from build123d import *

# Parameters (mm, degrees)
SKETCH_1_R          = 5
EXTRUDE_1_DEPTH     = 10
SKETCH_2_R          = 5
EXTRUDE_2_DEPTH     = 20
SKETCH_3_R          = 2.5
CUT_EXTRUDE_1_DEPTH = 15
SKETCH_4_R          = 2.5
CUT_EXTRUDE_2_DEPTH = 29.722813233


with BuildPart() as part:
    # 草圖1 → 填料-伸長1 (new, symmetric)
    with BuildSketch(Plane(origin=(0, 0, 0), x_dir=(1, 0, 0), z_dir=(0, 1, 0))):
        with Locations(Location((0, 0, 0), (0, 0, 270))):
            Circle(SKETCH_1_R)
    extrude(amount=EXTRUDE_1_DEPTH, both=True)

    # 草圖2 → 填料-伸長2 (add)
    with BuildSketch(Plane.XY):
        Circle(SKETCH_2_R)
    extrude(amount=EXTRUDE_2_DEPTH)

    # 草圖3 → 除料-伸長1 (cut)
    with BuildSketch(Plane.XY.offset(20)):
        Circle(SKETCH_3_R)
    extrude(amount=-CUT_EXTRUDE_1_DEPTH, mode=Mode.SUBTRACT)

    # 草圖4 → 除料-伸長2 (cut, through all)
    with BuildSketch(Plane.XZ.offset(10)):
        with Locations(Location((0, 0, 0), (0, 0, 270))):
            Circle(SKETCH_4_R)
    extrude(amount=-CUT_EXTRUDE_2_DEPTH, mode=Mode.SUBTRACT)


solid = part.part
Here's how the part is built. I have some questions about the finished solid (model axes, mm). A direction names the side the tool comes from. Coordinates: 2 decimals unless noted, no trailing zeros. Loops run counter-clockwise (first coordinate to the right, second up) from the corner with the lowest first, then second, coordinate; pieces in that order, holes last. Notation, with made-up numbers: (4.25, 54) -> (50.25, 54) arc R23 ccw to (50.25, 85) -> close; hole circle Ø9 at (63.25, 9). An arc over 180 degrees is marked (long way). Use one line per item in the form item = value. Start each with the question number.
(1) If we section it at B-B (y = 0): Please give me the cut outline in (x, z).
(2) If we section it at C-C (x = -3): Please give me the cut outline in (y, z).
(3) If we section it at D-D (z = 0.75): Please give me the cut outline in (x, y), then the cut area to 3 significant figures.
(4) If we section it at A-A (x = 0): Please give me the cut outline in (y, z), then the cut area to 3 significant figures.
(5) Will these pins go through, and if not, where does the flat tip stop? pin 1 (6 mm diameter, centred on y = -2, z = 11.5, fed in from +X); pin 2 (3 mm diameter, centred on x = 0, y = 0, fed in from +Z); pin 3 (1 mm diameter, centred on y = 3.5, z = 1.5, fed in from -X).
(6) On a 3-axis mill with a long thin cutter (end or side, diameter ignored), from which of +Z, -Z, +X, -X, +Y, -Y can I reach the whole of each face in a straight line? I mean faces 4 (the face through (-2, 10, 2)), 5 (the face through (0, 0, 5)). Say none if no direction works.
(7) Please list where these lines run through material, in increasing order: line 1 along X through (y, z) = (-4.5, 0); line 2 along Z through (x, y) = (1.5, 1); line 3 along Y through (x, z) = (2, 13.75).
(8) We'd pull the mould along Z, two halves only. Please class faces 1 (the face through (-2.44, -0.14, 0.54)), 2 (the face through (0, 0, -5)), 3 (the face through (-2, -10, 2)): pulls with the +Z half, pulls with the -Z half, needs draft (parallel to the pull), parting line crosses it, or undercut.
Verdict:
q1.outline = (-5, 0) arc R5 ccw to (5, 0) -> (5, 20) -> (2.5, 20) -> (2.5, 5) -> (-2.5, 5) -> (-2.5, 20) -> (-5, 20) -> close; hole circle Ø5 at (0, 0)
q2.outline = (-10, -4) -> (10, -4) -> (10, 4) -> (4, 4) -> (4, 20) -> (-4, 20) -> (-4, 4) -> (-10, 4) -> close
q3.outline = (-4.94, -10) -> (-2.38, -10) -> (-2.38, 10) -> (-4.94, 10) -> (-4.94, 0.75) arc R5 ccw to (-4.94, -0.75) -> close; (2.38, -10) -> (4.94, -10) -> (4.94, -0.75) arc R5 ccw to (4.94, 0.75) -> (4.94, 10) -> (2.38, 10) -> close
q3.area = 102 mm²
q4.outline = (-10, -5) -> (10, -5) -> (10, -2.5) -> (-10, -2.5) -> close; (-10, 2.5) -> (10, 2.5) -> (10, 5) -> (5, 5) -> (5, 20) -> (2.5, 20) -> (2.5, 5) -> (-2.5, 5) -> (-2.5, 20) -> (-5, 20) -> (-5, 5) -> (-10, 5) -> close
q4.area = 175 mm²
q5.pin_1 = 5
q5.pin_2 = 5
q5.pin_3 = -4.9
q6.face_4 = +Z, -Z, +X, -X, +Y
q6.face_5 = +Z
q7.line_1 = -5 to -2.5, 2.5 to 5
q7.line_2 = -4.77 to -2, 2 to 5
q7.line_3 = -4.58 to -1.5, 1.5 to 4.58
q8.face_1 = undercut
q8.face_2 = parting line crosses it
q8.face_3 = needs draft
